```python
from build123d import *

# Parameters (mm, degrees)
BOSS_EXTRUDE1_DEPTH = 2
SKETCH1_4_W         = 58.6
SKETCH1_4_H         = 54.7
BOSS_EXTRUDE2_DEPTH = 20


with BuildPart() as part:
    # Sketch1 → Boss-Extrude1 (new body)
    with BuildSketch(Plane(origin=(0, 0, 0), x_dir=(1, 0, 0), z_dir=(0, 1, 0))):
        Polygon((0, 0), (224.3, 0), (226.3, 0), (226.3, 58.7), (165.7, 58.7), (165.7, 69.2), (47.2, 69.2), (47.2, 81.5), (0, 81.5), align=None)
    extrude(amount=-BOSS_EXTRUDE1_DEPTH)

    # Sketch1<4> → Boss-Extrude2 (add)
    with BuildSketch(Plane(origin=(0, 0, 0), x_dir=(1, 0, 0), z_dir=(0, 1, 0))):
        Polygon((0, 2), (0, 0), (2, 0), (44.2, 0), (46.2, 0), (162.7, 0), (164.7, 0), (224.3, 0), (226.3, 0), (226.3, 58.7), (165.7, 58.7), (165.7, 69.2), (47.2, 69.2), (47.2, 81.5), (2, 81.5), (0, 81.5), (0, 79.5), align=None)
        Polygon((163.7, 2), (47.2, 2), (47.2, 67.2), (163.7, 67.2), (163.7, 55.7), (163.7, 53.7), align=None, mode=Mode.SUBTRACT)
        with Locations((195, 29.35)):
            Rectangle(SKETCH1_4_W, SKETCH1_4_H, mode=Mode.SUBTRACT)
        Polygon((2, 2), (2, 79.5), (45.2, 79.5), (45.2, 68.2), (45.2, 66.2), (45.2, 2), align=None, mode=Mode.SUBTRACT)
    extrude(amount=BOSS_EXTRUDE2_DEPTH)


solid = part.part
```
The model under review builds one solid part; all positions refer to its coordinate system, in mm. A direction names the side the tool comes from. Coordinates: 2 decimals unless noted, no trailing zeros. Write each loop counter-clockwise with the first axis right and the second up, starting at its lowest first coordinate (ties: lowest second). Pieces come first, ordered by that corner, then holes.
1) To check wall thickness, follow probe 1 along X at (y, z) = (6.5, -56); probe 2 along Z at (x, y) = (40.5, 1.5); probe 3 along Z at (x, y) = (183, 2.25). State the ranges of each line that lie inside material, in increasing order.
2) We need section A-A on y = 11.75. State the section outline as (x, z) points, then the cut area to 4 significant figures.
3) The part is to be moulded in two halves that separate along X. For faces 4 (the face through (0, 9, -41)), 5 (the face through (105, 0, -35)), 6 (the face through (107, 9, -69.2)), 7 (the face through (163.7, 10, -35)), say which applies: pulls with the +X half, pulls with the -X half, needs draft (parallel to the pull), parting line crosses it, or undercut.
4) Clearance check with flat-ended pins moving along their axes: pin 1 Ø3 at (x, y) = (100, 13) entering from +Z; pin 2 Ø3 at (y, z) = (13.5, -62) entering from +X; pin 3 Ø12 at (x, y) = (177.5, 17.5) entering from -Z; pin 4 Ø10 at (x, y) = (132, 13.5) entering from -Z. State where each tip first meets the part, or that it passes through.
5) We need section B-B on z = -11.5. State the section outline as (x, y) points, then the cut area to 3 significant figures.
6) We need section C-C on x = 65. State the section outline as (y, z) points.
7) Machinability: for faces 1 (the face through (195, 10, -2)), 2 (the face through (47.2, 9, -75)), 3 (the face through (112, 9, 0)), which of the approach directions +Z, -Z, +X, -X, +Y, -Y give a long, thin tool a straight path to every point of the face, cutting with its end or side? Answer none if there is none.
Answer list:
1. probe 1: x = 0 to 2, 45.2 to 47.2, 163.7 to 165.7, 224.3 to 226.3
1. probe 2: z = -81.5 to -79.5, -2 to 0
1. probe 3: z = -58.7 to -56.7, -2 to 0
2. outline: (0, -81.5) - (47.2, -81.5) - (47.2, -69.2) - (165.7, -69.2) - (165.7, -58.7) - (226.3, -58.7) - (226.3, 0) - (0, 0) - close; hole (2, -79.5) - (45.2, -79.5) - (45.2, -2) - (2, -2) - close; hole (47.2, -67.2) - (163.7, -67.2) - (163.7, -2) - (47.2, -2) - close; hole (165.7, -56.7) - (224.3, -56.7) - (224.3, -2) - (165.7, -2) - close
2. area: 1,455 mm2
3. face 4: pulls with the -X half
3. face 5: undercut
3. face 6: needs draft
3. face 7: undercut
4. pin 1: stops at z = 0
4. pin 2: stops at x = 165.7
4. pin 3: stops at z = -58.7
4. pin 4: stops at z = -69.2
5. outline: (0, -2) - (226.3, -2) - (226.3, 20) - (224.3, 20) - (224.3, 0) - (165.7, 0) - (165.7, 20) - (163.7, 20) - (163.7, 0) - (47.2, 0) - (47.2, 20) - (45.2, 20) - (45.2, 0) - (2, 0) - (2, 20) - (0, 20) - close
5. area: 613 mm2
6. outline: (-2, -69.2) - (20, -69.2) - (20, -67.2) - (0, -67.2) - (0, -2) - (20, -2) - (20, 0) - (-2, 0) - close
7. face 1: +Y
7. face 2: -Z, +X, +Y, -Y
7. face 3: +Z, +X, -X, +Y, -Y
